Check sheet for the modelled part. Datum: model origin and axes. Units: mm. Face numbers are marked on the shaded views. A direction names the side the tool comes from. Coordinates: 2 decimals unless noted, no trailing zeros. Write each loop counter-clockwise with the first axis right and the second up, starting at its lowest first coordinate (ties: lowest second). Pieces come first, ordered by that corner, then holes. Notation, with made-up numbers: (5, 13) - (61, 13) arc R23 ccw to (61, 34) - close; hole circle Ø3 at (21, -21). An arc over 180 degrees is marked (long way). Write each question's results on one line, items separated by ' | '.
from build123d import *

# Parameters (mm, degrees)
F0_W     = 381
F0_H     = 127
F1_DEPTH = 50.8
F2_W     = 368.3
F2_H     = 114.3
F3_DEPTH = 44.45
F4_R     = 3.175
F5_DEPTH = 6.351


with BuildPart() as f1:
    # F0 (on Front) → F1 (new body)
    with BuildSketch(Plane.XZ):
        with Locations((190.5, 63.5)):
            Rectangle(F0_W, F0_H)
    extrude(amount=-F1_DEPTH)

    # F2 (on face) → F3 (cut)
    with BuildSketch(Plane.XZ):
        with Locations((190.5, 63.5)):
            Rectangle(F2_W, F2_H)
    extrude(amount=-F3_DEPTH, mode=Mode.SUBTRACT)

    # F4 (on face) → F5 (cut, through all)
    with BuildSketch(Plane.XZ.offset(-44.45)):
        with Locations((53.955268, 63.5)):
            Circle(F4_R)
        with Locations((338.098884, 63.5)):
            Circle(F4_R)
    extrude(amount=-F5_DEPTH, mode=Mode.SUBTRACT)


solid = f1.part
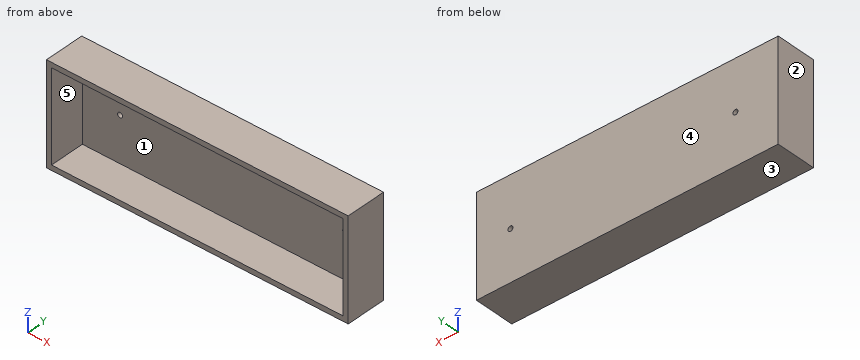
1. Sectioned sample at A-A (x = 261.5). Record the cut outline in (y, z), then the cut area to 3 significant figures.
Values follow:
outline: (0, 0) - (50.8, 0) - (50.8, 127) - (0, 127) - (0, 120.65) - (44.45, 120.65) - (44.45, 6.35) - (0, 6.35) - close | area: 1,370 mm^2
2. Material ranges on L1, parallel to X at y = 49, z = 63; L2, parallel to X at y = 35, z = 60; L3, parallel to Z at x = 35.5, y = 31, recorded low to high. Write a range as [from, to].
Values follow:
L1: x = [0, 50.82], [57.09, 334.96], [341.23, 381] | L2: x = [0, 6.35], [374.65, 381] | L3: z = [0, 6.35], [120.65, 127]
3. Sectioned sample at C-C (z = 52.5). Record the cut outline in (x, y).
Values follow:
outline: (0, 0) - (6.35, 0) - (6.35, 44.45) - (374.65, 44.45) - (374.65, 0) - (381, 0) - (381, 50.8) - (0, 50.8) - close
4. Draft check along Z on the marked faces 1, 2 and 3. Enter one of: pulls with the +Z half, pulls with the -Z half, needs draft (parallel to the pull), parting line crosses it, or undercut.
Values follow:
face 1: undercut | face 2: needs draft | face 3: pulls with the -Z half
5. Sectioned sample at B-B (y = 37). Record the cut outline in (x, z).
Values follow:
outline: (0, 0) - (381, 0) - (381, 127) - (0, 127) - close; hole (6.35, 6.35) - (374.65, 6.35) - (374.65, 120.65) - (6.35, 120.65) - close
6. Go/stop test with flat-tipped pins: pin 1 (1 mm diameter, centred on x = 194, z = 76, fed in from -Y); pin 2 (4 mm diameter, centred on x = 338.1, z = 63.5, fed in from -Y). Record where each tip stops, or that it passes through.
Values follow:
pin 1: stops at y = 44.45 | pin 2: passes through
7. Access from +Z, -Z, +X, -X, +Y, -Y to the whole of each face (thin tool, end or side, straight path). Record for the marked faces 4 and 5.
Values follow:
face 4: +Z, -Z, +X, -X, +Y | face 5: -Y
